Check sheet for the drawn part. Datum: minimum x, y, z corner. Units: mm. A direction names the side the tool comes from. Round coordinates to 2 decimals unless told otherwise and drop trailing zeros. Write each loop counter-clockwise with the first axis right and the second up, starting at its lowest first coordinate (ties: lowest second). Pieces come first, ordered by that corner, then holes. Notation, with made-up numbers: M 7,76.25 L 26,76.25 A7 ccw 26,81.25 Z; hole C 48,60 d8. An arc over 180 degrees is marked long. One line per item, written item: value.
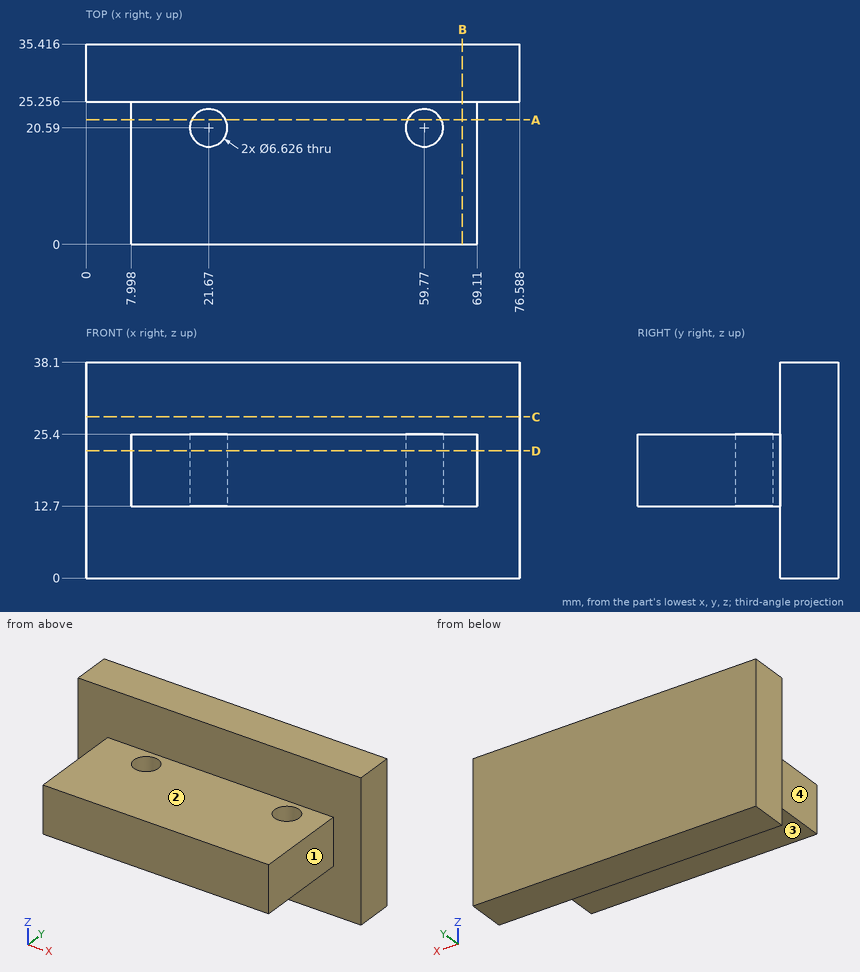
Q1. Depth check by flat-ended pin: P1, Ø4, axis at y = 9.5, z = 18.5, coming from the -X side; P2, Ø20, axis at x = 26, y = 9, coming from the +Z side; P3, Ø8.5, axis at x = 59.77, y = 20.59, coming from the -Z side; P4, Ø12, axis at y = 12.5, z = 32.5, coming from the -X side. Enter the tip coordinate at first touch or a pass-through.
Completed:
P1: x = 8
P2: z = 25.4
P3: z = 12.7
P4: through
Q2. Sectioned sample at B-B on x = 66.5. Enter the section's corners in (y, z), and give its area (3 significant figures).
Completed:
outline: M 0,12.7 L 25.26,12.7 L 25.26,0 L 35.42,0 L 35.42,38.1 L 25.26,38.1 L 25.26,25.4 L 0,25.4 Z
area: 708 mm^2
Q3. Access from +Z, -Z, +X, -X, +Y, -Y to the whole of each face (thin tool, end or side, straight path). Record for the marked faces 1, 2, 3 and 4.
Completed:
face 1: +Z, -Z, +X, -Y
face 2: +Z, +X, -X, -Y
face 3: -Z, +X, -X, -Y
face 4: +Z, -Z, -X, -Y
Q4. Scan lines: line 1 (Y direction, x = 8, z = 11); line 2 (Z direction, x = 31.5, y = 11.5); line 3 (X direction, y = 13, z = 16.5). Record each from-to range of solid material in increasing order. Write a range as [from, to].
Completed:
line 1: [25.26, 35.42]
line 2: [12.7, 25.4]
line 3: [8, 69.11]
Q5. Sectioned sample at A-A on y = 22. Enter the section's corners in (x, z), and give its area (3 significant figures).
Completed:
outline: M 8,12.7 L 18.67,12.7 L 18.67,25.4 L 8,25.4 Z; M 24.67,12.7 L 56.77,12.7 L 56.77,25.4 L 24.67,25.4 Z; M 62.77,12.7 L 69.11,12.7 L 69.11,25.4 L 62.77,25.4 Z
area: 624 mm^2
Q6. Sectioned sample at D-D on z = 22.5. Enter the section's corners in (x, y).
Completed:
outline: M 0,25.26 L 8,25.26 L 8,0 L 69.11,0 L 69.11,25.26 L 76.59,25.26 L 76.59,35.42 L 0,35.42 Z; hole C 21.67,20.59 d6.63; hole C 59.77,20.59 d6.63
Q7. Sectioned sample at C-C on z = 28.5. Enter the section's corners in (x, y).
Completed:
outline: M 0,25.26 L 76.59,25.26 L 76.59,35.42 L 0,35.42 Z
